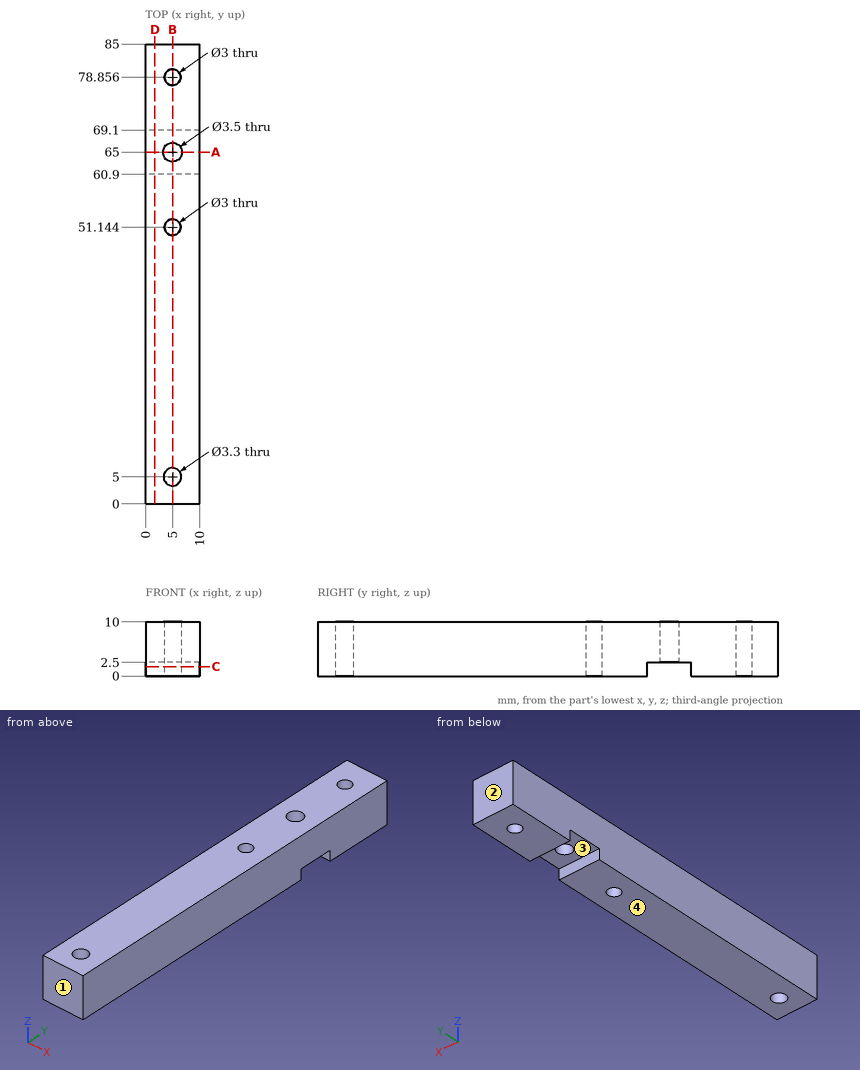
Job drawing, mm, ordinate dimensions from the low corner. One solid piece. Give positions to 0.01 mm unless a question says otherwise; leave off trailing zeros. Loops run counter-clockwise (first coordinate to the right, second up) from the corner with the lowest first, then second, coordinate; pieces in that order, holes last. Notation, with made-up numbers: M 57.25,6.25 L 110.25,6.25 A31 cw 110.25,38.25 Z; hole C 20.25,-28.75 d3. An arc over 180 degrees is marked long. Answer in a Markdown table with one row per item. Add a question column.
Item 1: Band-saw the part on C-C on z = 1.75. Give the cut face in (x, y), then the cut area to 3 significant figures.
Item 2: Band-saw the part on B-B on x = 5. Give the cut face in (y, z), then the cut area to 3 significant figures.
Item 3: Band-saw the part on D-D on x = 1.75. Give the cut face in (y, z), then the cut area to 4 significant figures.
Item 4: Mould opens along Y. For the marked faces 1, 2, 3 and 4 say: +Y half, -Y half, draft (parallel to the pull), parting line (faces both ways), or undercut.
Item 5: Probe probe 1 along Y at (x, z) = (5, 5.25); probe 2 along Y at (x, z) = (9.25, 1); probe 3 along Y at (x, z) = (6, 7). List the from-to ranges inside material, lowest first.
Item 6: Drop a flat-ended pin along its axis: P1, Ø2.5, axis at x = 4, y = 67, coming from the -Z side. Give the stop position or say it passes through.
Item 7: Band-saw the part on A-A on y = 65. Give the cut face in (x, z), then the cut area to 4 significant figures.
Reply:
| question | item | result |
|---|---|---|
| 1 | outline | M 0,0 L 10,0 L 10,60.9 L 0,60.9 Z; M 0,69.1 L 10,69.1 L 10,85 L 0,85 Z; hole C 5,5 d3.3; hole C 5,51.14 d3; hole C 5,78.86 d3 |
| 1 | area | 745 mm^2 |
| 2 | outline | M 0,0 L 3.35,0 L 3.35,10 L 0,10 Z; M 6.65,0 L 49.64,0 L 49.64,10 L 6.65,10 Z; M 52.64,0 L 60.9,0 L 60.9,2.5 L 63.25,2.5 L 63.25,10 L 52.64,10 Z; M 66.75,2.5 L 69.1,2.5 L 69.1,0 L 77.36,0 L 77.36,10 L 66.75,10 Z; M 80.36,0 L 85,0 L 85,10 L 80.36,10 Z |
| 2 | area | 710 mm^2 |
| 3 | outline | M 0,0 L 60.9,0 L 60.9,2.5 L 69.1,2.5 L 69.1,0 L 85,0 L 85,10 L 0,10 Z |
| 3 | area | 829.5 mm^2 |
| 4 | face 1 | -Y half |
| 4 | face 2 | +Y half |
| 4 | face 3 | undercut |
| 4 | face 4 | draft |
| 5 | probe 1 | y = 0 to 3.35, 6.65 to 49.64, 52.64 to 63.25, 66.75 to 77.36, 80.36 to 85 |
| 5 | probe 2 | y = 0 to 60.9, 69.1 to 85 |
| 5 | probe 3 | y = 0 to 3.69, 6.31 to 50.03, 52.26 to 63.56, 66.44 to 77.74, 79.97 to 85 |
| 6 | P1 | stops at z = 2.5 |
| 7 | outline | M 0,2.5 L 3.25,2.5 L 3.25,10 L 0,10 Z; M 6.75,2.5 L 10,2.5 L 10,10 L 6.75,10 Z |
| 7 | area | 48.75 mm^2 |
